Geometry: final body of the model. Coordinates: model frame, mm. A direction names the side the tool comes from. Give positions to 0.01 mm unless a question says otherwise; leave off trailing zeros. Loops run counter-clockwise (first coordinate to the right, second up) from the corner with the lowest first, then second, coordinate; pieces in that order, holes last.
1. Section C-C, the plane z = -12.5. Output: boundary loops of the cut face in (x, y).
2. Material intervals for line 1 along Z through (x, y) = (-25, 4.6); line 2 along X through (y, z) = (4.2, -12.5); line 3 along X through (y, z) = (5.1, -25), sorted ascending.
3. Section A-A, the plane y = 3.85. Output: boundary loops of the cut face in (x, z).
4. First-contact query: P1, Ø3.5, axis at x = -25, z = -37.5, coming from the -Y side; P2, Ø3, axis at x = -123.5, z = -12.5, coming from the +Y side. Flat tips, straight axial feed; report the tip coordinate or a pass-through.
5. Draft query along X for faces 3 (the face through (-122.09, 4.45, -13.42)), 4 (the face through (0, 3, -25)), 5 (the face through (-76, 3, -50)). Return one class per face: +X half, -X half, draft (parallel to the pull), parting line (faces both ways), or undercut.
6. Access query for faces 1 (the face through (-103.047, 4.446, -25.134)), 2 (the face through (-76, 0, -25)). Directions: +Z, -Z, +X, -X, +Y, -Y. A direction counts if a zero-diameter tool reaches every point of the face in a straight line with its end or side. Return the directions, or none.
7. Section B-B, the plane x = -75. Output: boundary loops of the cut face in (y, z).
8. Section D-D, the plane x = -25. Output: boundary loops of the cut face in (y, z).
from build123d import *

# Parameters (mm, degrees)
SKETCH1_W           = 150
SKETCH1_H           = 50
BOSS_EXTRUDE1_DEPTH = 5.95
SKETCH2_R           = 3.05
CUT_EXTRUDE1_DEPTH  = 3.05


with BuildPart() as part:
    # Sketch1 → Boss-Extrude1 (new body)
    with BuildSketch(Plane(origin=(0, 0, 0), x_dir=(1, 0, 0), z_dir=(0, 1, 0))):
        with Locations((-75, 25)):
            Rectangle(SKETCH1_W, SKETCH1_H)
    extrude(amount=BOSS_EXTRUDE1_DEPTH)

    # Sketch2 → Cut-Extrude1 (cut)
    with BuildSketch(Plane(origin=(0, 5.95, 0), x_dir=(1, 0, 0), z_dir=(0, 1, 0))):
        with Locations((-25, 37.5)):
            Circle(SKETCH2_R)
        with Locations((-25, 12.5)):
            Circle(SKETCH2_R)
        with Locations((-50, 25)):
            Circle(SKETCH2_R)
        with Locations((-75, 25)):
            Circle(SKETCH2_R)
        with Locations((-100, 25)):
            Circle(SKETCH2_R)
        with Locations((-125, 12.5)):
            Circle(SKETCH2_R)
        with Locations((-125, 37.5)):
            Circle(SKETCH2_R)
    extrude(amount=-CUT_EXTRUDE1_DEPTH, mode=Mode.SUBTRACT)


solid = part.part
Answers below:
1. outline: (-150, 0) - (0, 0) - (0, 5.95) - (-21.95, 5.95) - (-21.95, 2.9) - (-28.05, 2.9) - (-28.05, 5.95) - (-121.95, 5.95) - (-121.95, 2.9) - (-128.05, 2.9) - (-128.05, 5.95) - (-150, 5.95) - close
2. line 1: z = -50 to -40.55, -34.45 to -15.55, -9.45 to 0
2. line 2: x = -150 to -128.05, -121.95 to -28.05, -21.95 to 0
2. line 3: x = -150 to -103.05, -96.95 to -78.05, -71.95 to -53.05, -46.95 to 0
3. outline: (-150, -50) - (0, -50) - (0, 0) - (-150, 0) - close; hole circle Ø6.1 at (-125, -37.5); hole circle Ø6.1 at (-125, -12.5); hole circle Ø6.1 at (-100, -25); hole circle Ø6.1 at (-75, -25); hole circle Ø6.1 at (-50, -25); hole circle Ø6.1 at (-25, -37.5); hole circle Ø6.1 at (-25, -12.5)
4. P1: stops at y = 0
4. P2: stops at y = 2.9
5. face 3: undercut
5. face 4: +X half
5. face 5: draft
6. face 1: +Y
6. face 2: +Z, -Z, +X, -X, -Y
7. outline: (0, -50) - (5.95, -50) - (5.95, -28.05) - (2.9, -28.05) - (2.9, -21.95) - (5.95, -21.95) - (5.95, 0) - (0, 0) - close
8. outline: (0, -50) - (5.95, -50) - (5.95, -40.55) - (2.9, -40.55) - (2.9, -34.45) - (5.95, -34.45) - (5.95, -15.55) - (2.9, -15.55) - (2.9, -9.45) - (5.95, -9.45) - (5.95, 0) - (0, 0) - close
